Here's how the part is built. I have some questions about the finished solid (model axes, mm). Face numbers are marked on the shaded views. Round coordinates to 2 decimals unless told otherwise and drop trailing zeros. Loops run counter-clockwise (first coordinate to the right, second up) from the corner with the lowest first, then second, coordinate; pieces in that order, holes last. Notation, with made-up numbers: M 48,77.25 L 103,77.25 A8 cw 103,84.25 Z; hole C 41.25,-12.5 d3. An arc over 180 degrees is marked long. Answer as a JSON object with one key per item and string values.
from build123d import *

# Parameters (mm, degrees)
SKETCH1_R           = 36.25
SKETCH1_R_2         = 13.25
BOSS_EXTRUDE1_DEPTH = 20
BOSS_EXTRUDE3_START = 20
SKETCH2_R           = 36.25
SKETCH2_R_2         = 5.5
BOSS_EXTRUDE3_DEPTH = 20
SKETCH3_R           = 2.5
CUT_EXTRUDE1_DEPTH  = 66.024034018


with BuildPart() as part:
    # Sketch1 → Boss-Extrude1 (new body)
    with BuildSketch(Plane.XY):
        Circle(SKETCH1_R)
        Circle(SKETCH1_R_2, mode=Mode.SUBTRACT)
    extrude(amount=BOSS_EXTRUDE1_DEPTH)

    # Sketch2 → Boss-Extrude3 (add)
    with BuildSketch(Plane(origin=(0, 0, 0), x_dir=(-1, 0, 0), z_dir=(0, 0, -1)).offset(BOSS_EXTRUDE3_START)):
        Circle(SKETCH2_R)
        Circle(SKETCH2_R_2, mode=Mode.SUBTRACT)
    extrude(amount=-BOSS_EXTRUDE3_DEPTH)

    # Sketch3 → Cut-Extrude1 (cut, through all)
    with BuildSketch(Plane.XY.offset(20)):
        with Locations((-5.731515756, -29.447406119)):
            Circle(SKETCH3_R)
        with Locations((-22.636443897, 19.687341306)):
            Circle(SKETCH3_R)
        with Locations((28.367959653, 9.760064813)):
            Circle(SKETCH3_R)
    extrude(amount=-CUT_EXTRUDE1_DEPTH, mode=Mode.SUBTRACT)


solid = part.part
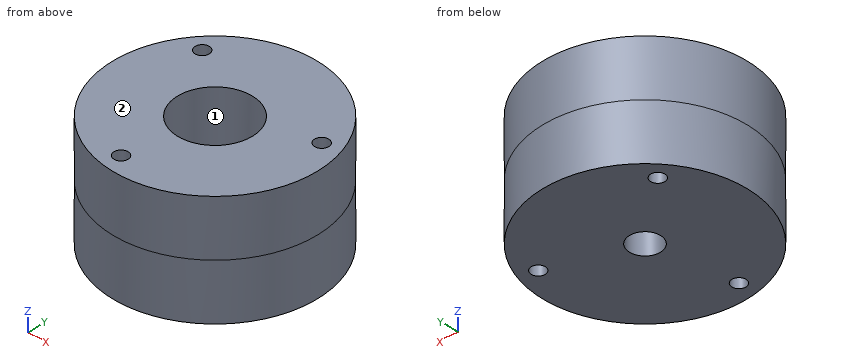
Item 1: Please list where these lines run through material, in increasing order: probe 1 along Y at (x, z) = (0, -15.75); probe 2 along Z at (x, y) = (-6, -2.5); probe 3 along Y at (x, z) = (2, -7). Write a range as from..to.
Resolved:
{"probe 1": "-36.25..-5.5, 5.5..36.25", "probe 2": "-20..0", "probe 3": "-36.19..-5.12, 5.12..36.19"}
Item 2: I want a section at A-A, the plane x = 0. Please give me the cut outline in (y, z), then the cut area to 3 significant figures.
Resolved:
{"outline": "M -36.25,-20 L -5.5,-20 L -5.5,0 L -13.25,0 L -13.25,20 L -36.25,20 Z; M 5.5,-20 L 36.25,-20 L 36.25,20 L 13.25,20 L 13.25,0 L 5.5,0 Z", "area": "2,150 mm²"}
Item 3: I'm going to push flat-ended pins straight in: pin 1 Ø4 at (x, z) = (-26.5, -11) entering from -Y; pin 2 Ø1.5 at (y, z) = (10, 0) entering from -X; pin 3 Ø14.5 at (x, y) = (0, 0) entering from +Z. Where does each tip first touch, or does it pass through?
Resolved:
{"pin 1": "y = -26.72", "pin 2": "x = -35.05", "pin 3": "z = 0"}
Item 4: If we mould it in two halves opening along X, with no side actions, what happens to the marked faces 1 and 2? For each: pulls with the +X half, pulls with the -X half, needs draft (parallel to the pull), parting line crosses it, or undercut.
Resolved:
{"face 1": "undercut", "face 2": "needs draft"}
Item 5: I want a section at D-D, the plane x = -10.5. Please give me the cut outline in (y, z).
Resolved:
{"outline": "M -34.7,-20 L 34.7,-20 L 34.7,20 L 8.08,20 L 8.08,0 L -8.08,0 L -8.08,20 L -34.7,20 Z"}
Item 6: I want a section at C-C, the plane z = 10.5. Please give me the cut outline in (x, y), then the cut area to 3 significant figures.
Resolved:
{"outline": "C 0,0 d72.5; hole C -22.64,19.69 d5; hole C 0,0 d26.5; hole C -5.73,-29.45 d5; hole C 28.37,9.76 d5", "area": "3,520 mm²"}
